from build123d import *

# Parameters (mm, degrees)
F0_W      = 266.7
F0_H      = 139.7
F1_DEPTH  = 7
F2_R      = 20
F3_R      = 62.5
F3_R_2    = 55.25
F4_DEPTH  = 3.5
F5_DEPTH  = 10
F6_R      = 3.25
F7_DEPTH  = 8
F8_R      = 2.5
F9_DEPTH  = 8
F10_R     = 5.625
F11_DEPTH = 2.8
F12_R     = 1.5
F13_R     = 3


with BuildPart() as f1:
    # F0 (on Top) → F1 (new body)
    with BuildSketch(Plane.XY):
        with Locations((70.65095, -0.318812)):
            Rectangle(F0_W, F0_H)
    extrude(amount=F1_DEPTH)

    # F2
    f2_edges = [f1.edges().sort_by_distance(p)[0] for p in [
        (-62.69905, 69.531188, 3.5),
        (204.00095, 69.531188, 3.5),
        (-62.69905, -70.168812, 3.5),
        (204.00095, -70.168812, 3.5),
    ]]
    fillet(f2_edges, radius=F2_R)

    # F3 (on face) → F4 (cut)
    with BuildSketch(Plane.XY.offset(7)):
        with Locations((66.581185, 0)):
            Circle(F3_R)
        with Locations((66.581185, 0)):
            Circle(F3_R_2, mode=Mode.SUBTRACT)
    extrude(amount=-F4_DEPTH, mode=Mode.SUBTRACT)

    # F3 (on face) → F5 (cut)
    with BuildSketch(Plane.XY.offset(7)):
        with Locations((66.581185, 0)):
            Circle(F3_R_2)
    extrude(amount=-F5_DEPTH, mode=Mode.SUBTRACT)

    # F6 (on face) → F7 (cut)
    with BuildSketch(Plane(origin=(0, 0, 0), x_dir=(1, 0, 0), z_dir=(0, 0, -1))):
        with Locations((-49.543765, 56.214787)):
            Circle(F6_R)
        with Locations((192.163914, 56.564152)):
            Circle(F6_R)
        with Locations((191.876724, -57.752054)):
            Circle(F6_R)
        with Locations((-49.089845, -57.752058)):
            Circle(F6_R)
    extrude(amount=-F7_DEPTH, mode=Mode.SUBTRACT)

    # F8 (on face) → F9 (cut)
    with BuildSketch(Plane.XY.offset(7)):
        with Locations((14.890482, 51.512826)):
            Circle(F8_R)
        with Locations((117.890482, 51.512826)):
            Circle(F8_R)
        with Locations((117.890482, -51.487174)):
            Circle(F8_R)
        with Locations((14.890482, -51.487174)):
            Circle(F8_R)
    extrude(amount=-F9_DEPTH, mode=Mode.SUBTRACT)

    # F10 (on face) → F11 (cut)
    with BuildSketch(Plane(origin=(0, 0, 0), x_dir=(1, 0, 0), z_dir=(0, 0, -1))):
        with Locations((14.890482, 51.487174)):
            Circle(F10_R)
        with Locations((117.890482, 51.487174)):
            Circle(F10_R)
        with Locations((117.890482, -51.512826)):
            Circle(F10_R)
        with Locations((14.890482, -51.512826)):
            Circle(F10_R)
    extrude(amount=-F11_DEPTH, mode=Mode.SUBTRACT)

    # F12
    f12_edges = [f1.edges().sort_by_distance(p)[0] for p in [
        (11.331185, 0, 0),
    ]]
    fillet(f12_edges, radius=F12_R)

    # F13
    f13_edges = [f1.edges().sort_by_distance(p)[0] for p in [
        (70.65095, 69.531188, 7),
    ]]
    fillet(f13_edges, radius=F13_R)


solid = f1.part
Geometry check sheet. Reference: the model listing, model coordinates, mm. A direction names the side the tool comes from. Round coordinates to 2 decimals unless told otherwise and drop trailing zeros. Loops run counter-clockwise (first coordinate to the right, second up) from the corner with the lowest first, then second, coordinate; pieces in that order, holes last.
Item 1: Access from +Z, -Z, +X, -X, +Y, -Y to the whole of each face (thin tool, end or side, straight path). Record for faces 5 (the flat face through (70.9, -55.3, 3.5)), 6 (the cylindrical face through (189.77, -58.76, 3.45)), 7 (the flat face through (120.3, 52.7, 2.8)).
Item 2: Mould release check, pull along X, two halves, no side actions. Record for faces 1 (the flat face through (98.4, 47.2, 0)), 2 (the cylindrical face through (-57, -64.15, 2.03)), 3 (the cylindrical face through (120.275, 52.264, 4.929)), 4 (the cylindrical face through (194.879, 58.997, 3.451)): pulls with the +X half, pulls with the -X half, needs draft (parallel to the pull), parting line crosses it, or undercut.
Item 3: Thickness scan on line 1 (X direction, y = 1.5, z = 1.5); line 2 (Z direction, x = 123.5, y = 17.5); line 3 (X direction, y = 16, z = 0.5). Record the ranges inside material, lowest first.
Item 4: Gauge pin test, flat ends, axial feed: pin 1 (5 mm diameter, centred on x = 192.16, y = -56.56, fed in from +Z); pin 2 (5.5 mm diameter, centred on x = 17, y = 52.5, fed in from -Z); pin 3 (3 mm diameter, centred on x = -10.5, y = -41.5, fed in from -Z). Record the tip position at first contact, or that the pin passes through.
Item 5: Cross-section at A-A on y = 0. Record the boundary of the cut face in (x, z), then the cut area to 3 significant figures.
Answer sheet:
1. face 5: +Z
1. face 6: +Z, -Z
1. face 7: -Z
2. face 1: needs draft
2. face 2: pulls with the -X half
2. face 3: undercut
2. face 4: undercut
3. line 1: x = -62.7 to 11.35, 121.81 to 204
3. line 2: z = 0 to 3.5
3. line 3: x = -62.7 to 13.3, 119.86 to 204
4. pin 1: passes through
4. pin 2: stops at z = 2.8
4. pin 3: stops at z = 0
5. outline: (-62.7, 0) - (9.83, 0) arc R1.5 ccw to (11.33, 1.5) - (11.33, 3.5) - (4.08, 3.5) - (4.08, 7) - (-59.7, 7) arc R3 ccw to (-62.7, 4) - close; (121.83, 1.5) arc R1.5 ccw to (123.33, 0) - (204, 0) - (204, 4) arc R3 ccw to (201, 7) - (129.08, 7) - (129.08, 3.5) - (121.83, 3.5) - close
5. area: 1,040 mm2
